from build123d import *

# Parameters (mm, degrees)
F0_W      = 148.8298028708
F0_H      = 94.5572704077
F1_DEPTH  = 67.818
F3_DEPTH  = 63.5
F4_W      = 77.2124454379
F4_H      = 15.4310404323
F5_DEPTH  = 100.33
F6_W      = 59.3081153929
F6_H      = 62.6651751809
F7_DEPTH  = 25.4
F8_W      = 29.6540576965
F8_H      = 6.8081544653
F9_DEPTH  = 87.122
F10_R     = 10.1527389167
F10_R_2   = 10.0169439882
F10_R_3   = 10.557482782
F10_R_4   = 10.2404194945
F11_DEPTH = 107.696


with BuildPart() as f1:
    # F0 (on Top) → F1 (new body)
    with BuildSketch(Plane.XY):
        Rectangle(F0_W, F0_H)
    extrude(amount=F1_DEPTH)

    # F2 (on Front) → F3 (cut, symmetric)
    with BuildSketch(Plane.XZ):
        Polygon((83.3928560285, 71.8970969319), (-11.1966025054, 71.8970969319), (83.3928560285, -10.0711896084), align=None)
    extrude(amount=F3_DEPTH, both=True, mode=Mode.SUBTRACT)

    # F4 (on face) → F5 (cut)
    with BuildSketch(Plane.XZ.offset(47.2786352038)):
        with Locations((-38.606222719, 2.9596809763)):
            Rectangle(F4_W, F4_H)
    extrude(amount=-F5_DEPTH, mode=Mode.SUBTRACT)

    # F6 (on face) → F7 (cut)
    with BuildSketch(Plane.XZ.offset(47.2786352038)):
        with Locations((43.6418186873, 26.5767483506)):
            Rectangle(F6_W, F6_H)
    extrude(amount=-F7_DEPTH, mode=Mode.SUBTRACT)

    # F8 (on face) → F9 (cut)
    with BuildSketch(Plane(origin=(-74.4149014354, 0, 0), x_dir=(0, -1, 0), z_dir=(-1, 0, 0))):
        with Locations((0, 67.818)):
            Rectangle(F8_W, F8_H)
    extrude(amount=-F9_DEPTH, mode=Mode.SUBTRACT)

    # F10 (on face) → F11 (cut)
    with BuildSketch(Plane(origin=(30.781032969, 0, 35.5205819779), x_dir=(0.7557256351, 0, -0.6548883603), z_dir=(0.6548883603, 0, 0.7557256351))):
        with Locations((-3.1062552259, -4.5893176019)):
            Circle(F10_R)
        with Locations((35.1240087858, -4.5893176019)):
            Circle(F10_R_2)
        with Locations((35.1240087858, 29.9893176019)):
            Circle(F10_R_3)
        with Locations((-3.1062552259, 29.9893176019)):
            Circle(F10_R_4)
    extrude(amount=-F11_DEPTH, mode=Mode.SUBTRACT)


solid = f1.part
Part model, mm, in its own coordinate system. A direction names the side the tool comes from. Give positions to 0.01 mm unless a question says otherwise; leave off trailing zeros. Write each loop counter-clockwise with the first axis right and the second up, starting at its lowest first coordinate (ties: lowest second). Pieces come first, ordered by that corner, then holes.
1) Probe L1, parallel to Y at x = 11.5, z = 22; L2, parallel to Y at x = 60, z = 8; L3, parallel to X at y = 27.5, z = 25.5. List the from-to ranges inside material, lowest first.
Resolved:
L1: y = -47.28 to -14.4, 5.22 to 20.09, 39.89 to 47.28
L2: y = -21.88 to -13.28, 4.1 to 20.68, 39.3 to 47.28
L3: x = -74.41 to 4.84, 31.13 to 42.34
2) Two-plate mould, pull along Z, no slides. Class faces 1 (the face through (-39, 14.827, 66)), 2 (the face through (-38, -1, 10.675)), 3 (the face through (11.6, -14.5, 21.5)): released by +Z, released by -Z, zero draft, split by the parting line, or undercut.
Resolved:
face 1: zero draft
face 2: released by -Z
face 3: undercut
3) Pin check, flat tips, straight feed: pin 1 (2.5 mm diameter, centred on y = 44.5, z = 7, fed in from -X); pin 2 (15 mm diameter, centred on x = -52.5, y = 1, fed in from +Z); pin 3 (6 mm diameter, centred on y = -3.5, z = 35.5, fed in from +X); pin 4 (8.5 mm diameter, centred on y = 9.5, z = 6.5, fed in from -X). Stop position of each tip, or through.
Resolved:
pin 1: stops at x = 0
pin 2: stops at z = 64.41
pin 3: stops at x = 15.96
pin 4: stops at x = -74.41
4) Cut at B-B on x = -52.5. Write the cut outline in (y, z).
Resolved:
outline: (-47.28, 10.68) - (47.28, 10.68) - (47.28, 67.82) - (14.83, 67.82) - (14.83, 64.41) - (-14.83, 64.41) - (-14.83, 67.82) - (-47.28, 67.82) - close
5) Cut at C-C on y = 37. Write the cut outline in (x, z), then the cut area to 3 significant figures.
Resolved:
outline: (-74.41, 10.68) - (-4.74, 10.68) - (22.79, 42.44) - (-6.49, 67.82) - (-74.41, 67.82) - close; (5.77, 0) - (36.03, 0) - (51.36, 17.69) - (34.07, 32.67) - close; (56.92, 0) - (71.77, 0) - (63.29, 7.35) - close
area: 5,560 mm2
6) Which spindle directions (+Z, -Z, +X, -X, +Y, -Y) get a long thin tool onto all of the face, cutting with end or side? Do faces 4 (the face through (0, -31, 5)), 5 (the face through (-39, -14.827, 66)), 6 (the face through (13.988, -35, 25)). Say none if no direction does.
Resolved:
face 4: -Z, -X, +Y, -Y
face 5: +Z, +X, -X
face 6: +Z, -Z, +X, -Y
7) Cut at D-D on z = 47. Write the cut outline in (x, y), then the cut area to 3 significant figures.
Resolved:
outline: (-74.41, -47.28) - (13.99, -47.28) - (13.99, -21.88) - (17.53, -21.88) - (17.53, 47.28) - (-74.41, 47.28) - close
area: 8,600 mm2
8) Cut at A-A on y = -17. Write the cut outline in (x, z).
Resolved:
outline: (-74.41, 10.68) - (0, 10.68) - (0, 0) - (71.77, 0) - (-6.49, 67.82) - (-74.41, 67.82) - close
